Work out the finished part from the listing and answer in its coordinate system (mm). A direction names the side the tool comes from. Round coordinates to 2 decimals unless told otherwise and drop trailing zeros. Loops run counter-clockwise (first coordinate to the right, second up) from the corner with the lowest first, then second, coordinate; pieces in that order, holes last. Notation, with made-up numbers: (-27.75, 42.25) - (-6.75, 42.25) arc R20 cw to (-6.75, 58.25) - close; hole circle Ø6 at (61.5, 0). An arc over 180 degrees is marked (long way). Return JSON: item names as keys, results as strings.
from build123d import *

# Parameters (mm, degrees)
F3_R      = 4.7
F4_DEPTH  = 29
F8_DEPTH  = 29
F6_R      = 4.7
F6_R_2    = 4
F9_DEPTH  = 10
F7_R      = 4.7
F7_R_2    = 4
F10_DEPTH = 12
F11_R     = 2.75
F12_DEPTH = 4.701


# Not quite as in the source:
# - ends of sketch curves that miss each other by under 0.0002 mm in the source are joined


with BuildPart() as f4:
    # F3 (on Front) → F4 (new body)
    with BuildSketch(Plane.XZ):
        Circle(F3_R)
    extrude(amount=F4_DEPTH)

    # F5 (on face) → F8 (cut, through all)
    with BuildSketch(Plane.XZ.offset(29)):
        with BuildLine():
            Line((-1.25, -3.8), (0, -3.8))
            Line((0, -3.8), (1.25, -3.8))
            Line((1.25, -3.8), (1.25, -3.7))
            ThreePointArc((1.25, -3.7), (1.3085786438, -3.5585786438), (1.45, -3.5))
            Line((1.45, -3.5), (2, -3.5))
            Line((2, -3.5), (2, -3.05))
            ThreePointArc((2, -3.05), (2.0585786438, -2.9085786438), (2.2, -2.85))
            Line((2.2, -2.85), (3.15, -2.85))
            Line((3.15, -2.85), (3.15, -2.15))
            Line((3.15, -2.15), (2.2, -2.15))
            ThreePointArc((2.2, -2.15), (2.0585786438, -2.0914213562), (2, -1.95))
            Line((2, -1.95), (2, -1.887459))
            ThreePointArc((2, -1.887459), (2.1033535752, -1.771554046), (2.2, -1.65))
            Line((2.2, -1.65), (3.75, -1.65))
            Line((3.75, -1.65), (3.75, 0))
            Line((3.75, 0), (3.75, 1.65))
            Line((3.75, 1.65), (2.2, 1.65))
            ThreePointArc((2.2, 1.65), (2.1033535752, 1.771554046), (1.9999998047, 1.8874588157))
            Line((1.9999998047, 1.8874588157), (2, 1.95))
            ThreePointArc((2, 1.95), (2.0585786438, 2.0914213562), (2.2, 2.15))
            Line((2.2, 2.15), (3.15, 2.15))
            Line((3.15, 2.15), (3.15, 2.85))
            Line((3.15, 2.85), (2.2, 2.85))
            ThreePointArc((2.2, 2.85), (2.0585786438, 2.9085786438), (2, 3.05))
            Line((2, 3.05), (2, 3.5))
            Line((2, 3.5), (1.45, 3.5))
            ThreePointArc((1.45, 3.5), (1.3085786438, 3.5585786438), (1.25, 3.7))
            Line((1.25, 3.7), (1.25, 3.8))
            Line((1.25, 3.8), (0, 3.8))
            Line((0, 3.8), (-1.25, 3.8))
            Line((-1.25, 3.8), (-1.25, 3.7))
            ThreePointArc((-1.25, 3.7), (-1.3085786438, 3.5585786438), (-1.45, 3.5))
            Line((-1.45, 3.5), (-2, 3.5))
            Line((-2, 3.5), (-2, 3.05))
            ThreePointArc((-2, 3.05), (-2.0585786438, 2.9085786438), (-2.2, 2.85))
            Line((-2.2, 2.85), (-3.15, 2.85))
            Line((-3.15, 2.85), (-3.15, 2.15))
            Line((-3.15, 2.15), (-2.2, 2.15))
            ThreePointArc((-2.2, 2.15), (-2.0585786438, 2.0914213562), (-2, 1.95))
            Line((-2, 1.95), (-2, 1.887459))
            ThreePointArc((-2, 1.887459), (-2.1033535752, 1.771554046), (-2.2, 1.65))
            Line((-2.2, 1.65), (-3.75, 1.65))
            Line((-3.75, 1.65), (-3.75, 0))
            Line((-3.75, 0), (-3.75, -1.65))
            Line((-3.75, -1.65), (-2.2, -1.65))
            ThreePointArc((-2.2, -1.65), (-2.1033535752, -1.771554046), (-1.9999998047, -1.8874588157))
            Line((-1.9999998047, -1.8874588157), (-2, -1.95))
            ThreePointArc((-2, -1.95), (-2.0585786438, -2.0914213562), (-2.2, -2.15))
            Line((-2.2, -2.15), (-3.15, -2.15))
            Line((-3.15, -2.15), (-3.15, -2.85))
            Line((-3.15, -2.85), (-2.2, -2.85))
            ThreePointArc((-2.2, -2.85), (-2.0585786438, -2.9085786438), (-2, -3.05))
            Line((-2, -3.05), (-2, -3.5))
            Line((-2, -3.5), (-1.45, -3.5))
            ThreePointArc((-1.45, -3.5), (-1.3085786438, -3.5585786438), (-1.25, -3.7))
            Line((-1.25, -3.7), (-1.25, -3.8))
        make_face()
    extrude(amount=-F8_DEPTH, mode=Mode.SUBTRACT)

    # F6 (on face) → F9 (join)
    with BuildSketch(Plane.XZ.offset(29)):
        Circle(F6_R)
        Circle(F6_R_2, mode=Mode.SUBTRACT)
    extrude(amount=F9_DEPTH)

    # F7 (on face) → F10 (join)
    with BuildSketch(Plane(origin=(0, 0, 0), x_dir=(-1, 0, 0), z_dir=(0, 1, 0))):
        Circle(F7_R)
        Circle(F7_R_2, mode=Mode.SUBTRACT)
    extrude(amount=F10_DEPTH)

    # F11 (on Right) → F12 (cut, through all)
    with BuildSketch(Plane.YZ):
        with Locations((-32.75, 0)):
            Circle(F11_R)
    extrude(amount=-F12_DEPTH, mode=Mode.SUBTRACT)


solid = f4.part
1) Flat-ended cylindrical pins translate along their axes: pin 1 (1 mm diameter, centred on y = -18.5, z = -1, fed in from +X); pin 2 (2 mm diameter, centred on y = -33, z = 3.5, fed in from +X); pin 3 (1 mm diameter, centred on x = 3, z = -1.5, fed in from -Y). Find the tip coordinate at first contact, or state that the pin passes through.
Verdict:
{"pin 1": "stops at x = 4.67", "pin 2": "stops at x = 3.98", "pin 3": "stops at y = -29"}
2) Determine the mould class of faces 1 (the flat face through (2.81, -29, -1.96)), 2 (the flat face through (-2, 12, 4)), 3 (the cylindrical face through (0.867, 5.916, -3.905)) for opening direction Z: pulls with the +Z half, pulls with the -Z half, needs draft (parallel to the pull), parting line crosses it, or undercut.
Verdict:
{"face 1": "undercut", "face 2": "needs draft", "face 3": "undercut"}
3) Section B-B (z = 0) is taken. Give the vertices of the cut face in (x, y), and give its area (4 significant figures).
Verdict:
{"outline": "(-4.7, -39) - (-4, -39) - (-4, -35.5) - (-4.7, -35.5) - close; (-4.7, -30) - (-4, -30) - (-4, -29) - (-3.75, -29) - (-3.75, 0) - (-4, 0) - (-4, 12) - (-4.7, 12) - close; (3.75, -29) - (4, -29) - (4, -39) - (4.7, -39) - (4.7, 12) - (4, 12) - (4, 0) - (3.75, 0) - close", "area": "82.05 mm2"}
4) Section A-A (x = 0) is taken. Give the vertices of the cut face in (y, z).
Verdict:
{"outline": "(-39, -4.7) - (12, -4.7) - (12, -4) - (0, -4) - (0, -3.8) - (-29, -3.8) - (-29, -4) - (-39, -4) - close; (-39, 4) - (-29, 4) - (-29, 3.8) - (0, 3.8) - (0, 4) - (12, 4) - (12, 4.7) - (-39, 4.7) - close"}
5) A tool of negligible diameter and unlimited length cuts with its end or side. For faces 4 (the flat face through (-2.83, -29, -1.96)), 5 (the flat face through (-3.75, -15, 0)), 6 (the cylindrical face through (-4.19, -30.13, 0.83)), from which of +Z, -Z, +X, -X, +Y, -Y can it reach the whole face along a straight path? Write none if from no direction.
Verdict:
{"face 4": "-Y", "face 5": "none", "face 6": "-X"}
6) Section D-D (y = -32.75) is taken. Give the vertices of the cut face in (x, z), and give its area (3 significant figures).
Verdict:
{"outline": "(-3.81, -2.75) arc R4.7 ccw (long way) to (-3.81, 2.75) - (-2.9, 2.75) arc R4 cw (long way) to (-2.9, -2.75) - close", "area": "15.0 mm2"}
7) Section C-C (y = 8) is taken. Give the vertices of the cut face in (x, z), and give its area (3 significant figures).
Verdict:
{"outline": "circle Ø9.4 at (0, 0); hole circle Ø8 at (0, 0)", "area": "19.1 mm2"}
8) Find the intervals of material crossed by L1, parallel to X at y = -19.5, z = 2.75; L2, parallel to Z at x = -2.25, y = -9.5; L3, parallel to Z at x = 0, y = 8.5, in increasing order.
Verdict:
{"L1": "x = -3.81 to -3.15, 3.15 to 3.81", "L2": "z = -4.13 to -2.85, -2.15 to -1.65, 1.65 to 2.15, 2.85 to 4.13", "L3": "z = -4.7 to -4, 4 to 4.7"}
